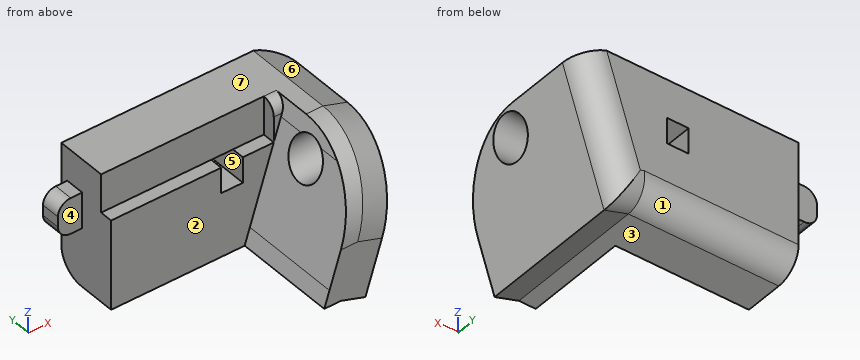
```python
from build123d import *

# Parameters (mm, degrees)
BOSS_EXTRUDE1_DEPTH     = 33.02
CUT_EXTRUDE1_DEPTH      = 20.32
FILLET1_R               = 15.24
SKETCH4_W               = 4.318
SKETCH4_H               = 5.08
CUT_EXTRUDE3_DEPTH      = 20.32
FILLET2_R               = 2.54
BOSS_EXTRUDE2_DEPTH     = 5.08
BOSS_EXTRUDE3_DEPTH     = 5.08
CUT_EXTRUDE2_DEPTH      = 88.392
CUT_EXTRUDE2_DEPTH_BACK = 20.32
SKETCH3_R               = 4.064
FILLET3_R               = 5.08
SKETCH7_W               = 44.236060242
SKETCH7_H               = 34.660368577
CUT_EXTRUDE4_DEPTH      = 37.084
SKETCH8_W               = 7.112
SKETCH8_H               = 3.81
BOSS_EXTRUDE4_DEPTH     = 4.826
FILLET4_R               = 2.54
SKETCH9_W               = 32.557227401
SKETCH9_H               = 7.62
CUT_EXTRUDE5_DEPTH      = 2.54


with BuildPart() as part:
    # Sketch1 → Boss-Extrude1 (new body)
    with BuildSketch(Plane(origin=(0, 0, 0), x_dir=(1, 0, 0), z_dir=(0, 1, 0))):
        Polygon((0, 0), (-8.252960284, -25.4), (67.947039716, -25.4), (59.694079431, 0), align=None)
    extrude(amount=BOSS_EXTRUDE1_DEPTH)

    # Sketch2 → Cut-Extrude1 (cut)
    with BuildSketch(Plane.XZ):
        Polygon((-3.882947687, 22.225), (-6.015103815, 28.787101815), (66.521112465, 31.285963003), (63.577027118, 22.225), (57.387306905, 3.175), (55.156358593, -3.691152891), (4.897822181, -4.799430866), (2.306772526, 3.175), align=None)
    extrude(amount=-CUT_EXTRUDE1_DEPTH, mode=Mode.SUBTRACT)

    # Fillet1
    # the kernel refuses this fillet: 15.24 mm, written as the material it takes off along each edge
    with BuildSketch(Plane(origin=(26.508647154, 0, 25.4), x_dir=(0, 1, 0), z_dir=(1, 0, 0)), Plane(origin=(-46.352960284, 0, 25.4), x_dir=(0, 1, 0), z_dir=(1, 0, 0))) as fillet1_piece_1:
        with BuildLine():
            CenterArc((FILLET1_R, -FILLET1_R), FILLET1_R, 90, 90)
            Line((0, -FILLET1_R), (0, 0))
            Line((0, 0), (FILLET1_R, 0))
        make_face()
    extrude(amount=79.538392562, mode=Mode.SUBTRACT)

    # Sketch4 → Cut-Extrude3 (cut)
    with BuildSketch(Plane(origin=(0, 33.02, 0), x_dir=(1, 0, 0), z_dir=(0, 1, 0))):
        with Locations((53.850039716, -15.24)):
            Rectangle(SKETCH4_W, SKETCH4_H)
        with Locations((5.844039716, -15.24)):
            Rectangle(SKETCH4_W, SKETCH4_H)
    extrude(amount=-CUT_EXTRUDE3_DEPTH, mode=Mode.SUBTRACT)

    # Fillet2
    fillet2_edges = [part.edges().sort_by_distance(p)[0] for p in [
        (29.847039716, 20.32, 25.4),
    ]]
    fillet(fillet2_edges, radius=FILLET2_R)

    # Sketch5 → Boss-Extrude2 (add)
    with BuildSketch(Plane(origin=(0, 0, 0), x_dir=(-0.3090169943749446, 0, 0.9510565162951545), z_dir=(-0.9510565162951545, 0, -0.3090169943749446))):
        with BuildLine():
            Line((0, 0), (10.682856198, 0))
            add(Edge.make_bspline(
                [(10.682856198, 0), (26.707140496, 0), (26.707140496, 15.24)],
                knots=[1.570796327, 1.570796327, 1.570796327, 3.141592654, 3.141592654, 3.141592654], degree=2, weights=[1, 0.707106781, 1]))
            Line((26.707140496, 15.24), (26.707140496, 33.02))
            Line((26.707140496, 33.02), (0, 33.02))
            Line((0, 33.02), (0, 0))
        make_face()
    extrude(amount=BOSS_EXTRUDE2_DEPTH)

    # Sketch6 → Boss-Extrude3 (add)
    with BuildSketch(Plane(origin=(53.993802077, 0, -17.543649769), x_dir=(-0.30901699437494445, 0, -0.9510565162951545), z_dir=(0.9510565162951545, 0, -0.30901699437494445))):
        with BuildLine():
            Line((-45.153625504, 33.02), (-45.153625504, 15.24))
            add(Edge.make_bspline(
                [(-45.153625504, 15.24), (-45.153625504, 0), (-29.129341206, 0)],
                knots=[0, 0, 0, 1.570796327, 1.570796327, 1.570796327], degree=2, weights=[1, 0.707106781, 1]))
            Line((-29.129341206, 0), (-18.446485008, 0))
            Line((-18.446485008, 0), (-18.446485008, 33.02))
            Line((-18.446485008, 33.02), (-45.153625504, 33.02))
        make_face()
    extrude(amount=BOSS_EXTRUDE3_DEPTH)

    # Sketch3 → Cut-Extrude2 (cut, two sides: drawn at the far end of the back side and taken through both)
    with BuildSketch(Plane(origin=(0, 0, 0), x_dir=(0, 0, -1), z_dir=(1, 0, 0)).offset(-CUT_EXTRUDE2_DEPTH_BACK)):
        with Locations((-19.05, 12.7)):
            Circle(SKETCH3_R)
    extrude(amount=CUT_EXTRUDE2_DEPTH + CUT_EXTRUDE2_DEPTH_BACK, mode=Mode.SUBTRACT)

    # Fillet3
    fillet3_edges = [part.edges().sort_by_distance(p)[0] for p in [
        (-2.415683551, 33.02, -0.784903166),
        (62.109762983, 33.02, -0.784903166),
        (29.847039716, 33.02, 0),
        (-8.957847245, 33.02, 11.130193669),
        (68.651926676, 33.02, 11.130193669),
    ]]
    fillet(fillet3_edges, radius=FILLET3_R)

    # Sketch7 → Cut-Extrude4 (cut)
    with BuildSketch(Plane(origin=(0, 33.02, 0), x_dir=(1, 0, 0), z_dir=(0, 1, 0))):
        with Locations((7.729009595, -8.069815712)):
            Rectangle(SKETCH7_W, SKETCH7_H)
    extrude(amount=-CUT_EXTRUDE4_DEPTH, mode=Mode.SUBTRACT)

    # Sketch8 → Boss-Extrude4 (add)
    with BuildSketch(Plane.ZY.offset(-29.847039716)):
        with Locations((15.24, 29.591)):
            Rectangle(SKETCH8_W, SKETCH8_H)
    extrude(amount=BOSS_EXTRUDE4_DEPTH)

    # Fillet4
    fillet4_edges = [part.edges().sort_by_distance(p)[0] for p in [
        (25.021039716, 29.591, 18.796),
        (25.021039716, 29.591, 11.684),
    ]]
    fillet(fillet4_edges, radius=FILLET4_R)

    # Sketch9 → Cut-Extrude5 (cut)
    with BuildSketch(Plane.XZ.offset(-20.32)):
        with Locations((45.854145368, 21.59)):
            Rectangle(SKETCH9_W, SKETCH9_H)
    extrude(amount=-CUT_EXTRUDE5_DEPTH, mode=Mode.SUBTRACT)


solid = part.part
```
Part model, mm, in its own coordinate system. Face numbers are marked on the shaded views. A direction names the side the tool comes from. Round coordinates to 2 decimals unless told otherwise and drop trailing zeros. Loops run counter-clockwise (first coordinate to the right, second up) from the corner with the lowest first, then second, coordinate; pieces in that order, holes last. Notation, with made-up numbers: (64.5, -11.5) -> (91.5, -11.5) arc R30 cw to (91.5, 10.5) -> close; hole circle Ø1 at (43, 40). An arc over 180 degrees is marked (long way). Use a Markdown table: item, result.
1) Probe line 1 (Z direction, x = 53, y = 24.5); line 2 (Y direction, x = 66, z = 19.05); line 3 (Y direction, x = 42, z = 11). List the from-to ranges inside material, lowest first. Write a range as [from, to].
The answers:
| item | result |
|---|---|
| line 1 | z = [0, 12.7], [17.78, 25.4] |
| line 2 | y = [2.89, 8.64], [16.76, 33.02] |
| line 3 | y = [20.32, 33.02] |
2) Cut at A-A, the plane y = 23.5. List the corners of the cut face in (x, z).
The answers:
| item | result |
|---|---|
| outline | (29.85, 0) -> (59.69, 0) -> (64.53, -1.57) -> (72.78, 23.83) -> (67.95, 25.4) -> (29.85, 25.4) -> close; hole (51.69, 12.7) -> (56.01, 12.7) -> (56.01, 17.78) -> (51.69, 17.78) -> close |
3) Cut at B-B, the plane x = 47.5. List the corners of the cut face in (y, z).
The answers:
| item | result |
|---|---|
| outline | (20.32, 0) -> (27.94, 0) arc R5.08 ccw to (33.02, 5.08) -> (33.02, 25.4) -> (22.86, 25.4) -> (22.86, 17.78) -> (20.32, 17.78) -> close |
4) Tool access for the marked faces 1, 2, 3 and 4: list every direction of +Z, -Z, +X, -X, +Y, -Y with a clear straight run to the whole face (end or side of a thin tool).
The answers:
| item | result |
|---|---|
| face 1 | -Z, -X, +Y |
| face 2 | +Z, -X, -Y |
| face 3 | -Z, -X, +Y, -Y |
| face 4 | +Z, -Z, -X, -Y |
5) Pull direction X, two halves, no side cores. Call the marked faces 5, 6 and 7: pulls with the +X half, pulls with the -X half, needs draft (parallel to the pull), parting line crosses it, or undercut.
The answers:
| item | result |
|---|---|
| face 5 | undercut |
| face 6 | pulls with the +X half |
| face 7 | needs draft |
6) Drop flat-ended pins along their axis: pin 1 Ø2.5 at (x, z) = (28, 14.5) entering from -Y; pin 2 Ø3 at (x, y) = (44, 22) entering from +Z; pin 3 Ø1 at (x, z) = (37.5, 2.5) entering from -Y; pin 4 Ø5 at (y, z) = (22, 13.5) entering from -X. Give the stop position or say it passes through.
The answers:
| item | result |
|---|---|
| pin 1 | stops at y = 27.69 |
| pin 2 | stops at z = 25.4 |
| pin 3 | stops at y = 20.32 |
| pin 4 | stops at x = 29.85 |
